Geometry: final body of the model. Coordinates: model frame, mm. Face numbers are marked on the shaded views. Coordinates: 2 decimals unless noted, no trailing zeros. Loops run counter-clockwise (first coordinate to the right, second up) from the corner with the lowest first, then second, coordinate; pieces in that order, holes last. Notation, with made-up numbers: (14, 6.5) -> (34, 6.5) arc R8 ccw to (34, 12.5) -> close; hole circle Ø2 at (-11, 23). An arc over 180 degrees is marked (long way). One line per item, written item: value. Start each with the question number.
Item 1: Section query A-A on y = 0. Return loops of the section in (x, z).
Item 2: Ray query, probe 1 along Y at (x, z) = (52.5, 4); probe 2 along Z at (x, y) = (61.5, 2.5); probe 3 along Y at (x, z) = (71.5, 4). Return the intervals inside material, ascending. Write a range as from..to.
Item 3: Section query D-D on x = 97.5. Return loops of the section in (y, z), then the cut area to 3 significant figures.
Item 4: Mould query, pull axis Z, two halves, no side actions, for the marked faces 1 and 2. Classes: +Z half, -Z half, draft (parallel to the pull), parting line (faces both ways), or undercut.
Item 5: Contact query for flat-ended pins moving along their axis: pin 1 Ø3 at (x, z) = (102.5, -21) entering from +Y; pin 2 Ø18 at (y, z) = (0, 0) entering from -X; pin 3 Ø5 at (y, z) = (11, 14) entering from +X. Output: stop coordinate, or through.
Item 6: Section query C-C on x = 36. Return loops of the section in (y, z), then the cut area to 3 significant figures.
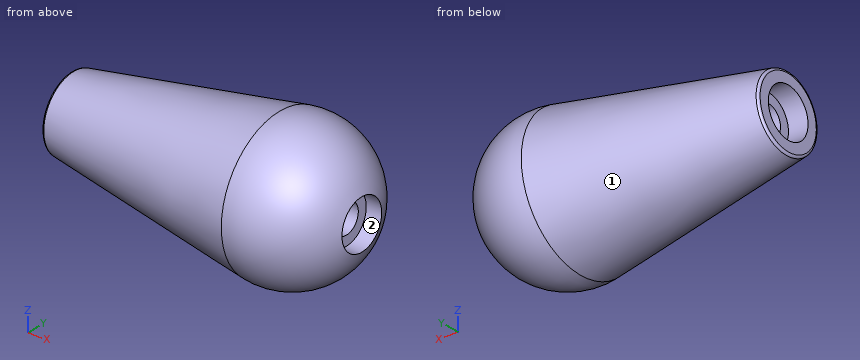
from build123d import *

# Parameters (mm, degrees)
FILLET1_R = 1


with BuildPart() as part:
    # Sketch1 → Revolve1 (revolve)
    with BuildSketch(Plane(origin=(0, 0, 0), x_dir=(1, 0, 0), z_dir=(0, 1, 0))):
        with BuildLine():
            Line((0, 0), (120, 0))
            ThreePointArc((120, 0), (109.337020363, 22.936426127), (84.928023767, 29.568142605))
            Line((84.928023767, 29.568142605), (0, 15))
            Line((0, 15), (0, 0))
        make_face()
    revolve(axis=Axis((0, 0, 0), (1, 0, 0)))

    # Sketch2 → Cut-Revolve2 (revolve, cut)
    with BuildSketch(Plane.XY, mode=Mode.PRIVATE) as cut_revolve2_sk:
        Polygon((0, 0), (120, 0), (120, 10), (112, 10), (112, 6), (8, 6), (8, 10), (0, 10), align=None)
    revolve(cut_revolve2_sk.sketch.rotate(Axis((0, 0, 0), (1, 0, 0)), 180), axis=Axis((0, 0, 0), (1, 0, 0)), mode=Mode.SUBTRACT)

    # Fillet1
    fillet1_edges = [part.edges().sort_by_distance(p)[0] for p in [
        (0, 0, 15),
    ]]
    fillet(fillet1_edges, radius=FILLET1_R)


solid = part.part
Reply:
1. outline: (0, -14.16) arc R1 ccw to (0.83, -15.14) -> (84.93, -29.57) arc R30 ccw to (118.28, -10) -> (112, -10) -> (112, -6) -> (8, -6) -> (8, -10) -> (0, -10) -> close; (0, 10) -> (8, 10) -> (8, 6) -> (112, 6) -> (112, 10) -> (118.28, 10) arc R30 ccw to (84.93, 29.57) -> (0.83, 15.14) arc R1 ccw to (0, 14.16) -> close
2. probe 1: y = -23.67..-4.47, 4.47..23.67
2. probe 2: z = -25.43..-5.45, 5.45..25.43
2. probe 3: y = -26.97..-4.47, 4.47..26.97
3. outline: circle Ø58.09 at (0, 0); hole circle Ø12 at (0, 0)
3. area: 2,540 mm²
4. face 1: parting line
4. face 2: undercut
5. pin 1: stops at y = 19.33
5. pin 2: stops at x = 8
5. pin 3: stops at x = 115.8
6. outline: circle Ø42.35 at (0, 0); hole circle Ø12 at (0, 0)
6. area: 1,300 mm²
